```python
from build123d import *

# Parameters (mm, degrees)
SKETCH1_W            = 128
SKETCH1_H            = 85.7
BOSS_EXTRUDE1_DEPTH  = 3
M6_CLEARANCE_HOLE1_D = 6.6
FILLET1_R            = 3


with BuildPart() as part:
    # Sketch1 → Boss-Extrude1 (new body)
    with BuildSketch(Plane(origin=(0, 0, 0), x_dir=(1, 0, 0), z_dir=(0, 1, 0))):
        Rectangle(SKETCH1_W, SKETCH1_H)
    extrude(amount=BOSS_EXTRUDE1_DEPTH)

    # M6 Clearance Hole1 (through all)
    with Locations(Plane(origin=(0, 3, 0), x_dir=(1, 0, 0), z_dir=(0, 1, 0))):
        with Locations((-60.5, 39.35), (0, 39.35), (60.5, 39.35), (60.5, 0), (60.5, -39.35), (0, -39.35), (-60.5, -39.35), (-60.5, 0), (0, -20.01), (0, 20.01)):
            Hole(M6_CLEARANCE_HOLE1_D / 2)

    # Fillet1
    fillet1_edges = [part.edges().sort_by_distance(p)[0] for p in [
        (64, 1.5, 42.85),
        (-64, 1.5, 42.85),
        (-64, 1.5, -42.85),
        (64, 1.5, -42.85),
    ]]
    fillet(fillet1_edges, radius=FILLET1_R)


solid = part.part
```
Read the model definition and answer for the solid it produces. Units are mm, in the model's axes. Give positions to 0.01 mm unless a question says otherwise; leave off trailing zeros. Write each loop counter-clockwise with the first axis right and the second up, starting at its lowest first coordinate (ties: lowest second). Pieces come first, ordered by that corner, then holes. Notation, with made-up numbers: M 78.5,80.25 L 96.5,80.25 A24 ccw 96.5,98.25 Z; hole C 87,50 d8. An arc over 180 degrees is marked long. Put each result on its own line as item: value. Start each with the question number.
1. The part is cut by section A-A, the plane z = 0. Give the vertices of the cut face in (x, y), and give its area (3 significant figures).
2. The part is cut by section C-C, the plane x = 0. Give the vertices of the cut face in (y, z), and give its area (3 significant figures).
3. Consider line 1 along Z through (x, y) = (0, 1.1); line 2 along X through (y, z) = (1.3, -39.35); line 3 along Z through (x, y) = (-60.5, 1.55). Determine where each line is inside the solid, lowest interval first.
4. The part is cut by section B-B, the plane z = 20.01. Give the vertices of the cut face in (x, y).
5. For a pull along X with two mould halves and no side action, classify faces 1 (the cylindrical face through (-63.14, 1.52, -41.95)), 2 (the cylindrical face through (0.72, 1.48, 42.57)), 3 (the cylindrical face through (0.43, 1.48, -42.62)), 4 (the cylindrical face through (63.1, 1.52, 41.99)) as released by +X, released by -X, zero draft, split by the parting line, or undercut.
6. The part is cut by section D-D, the plane y = 1.65. Give the number of separate pieces and of enclosed holes in the cut face, and give its area (3 significant figures).
Final values:
1. outline: M -64,0 L -63.8,0 L -63.8,3 L -64,3 Z; M -57.2,0 L 57.2,0 L 57.2,3 L -57.2,3 Z; M 63.8,0 L 64,0 L 64,3 L 63.8,3 Z
1. area: 344 mm²
2. outline: M 0,-42.85 L 3,-42.85 L 3,-42.65 L 0,-42.65 Z; M 0,-36.05 L 3,-36.05 L 3,-23.31 L 0,-23.31 Z; M 0,-16.71 L 3,-16.71 L 3,16.71 L 0,16.71 Z; M 0,23.31 L 3,23.31 L 3,36.05 L 0,36.05 Z; M 0,42.65 L 3,42.65 L 3,42.85 L 0,42.85 Z
2. area: 178 mm²
3. line 1: z = -42.85 to -42.65, -36.05 to -23.31, -16.71 to 16.71, 23.31 to 36.05, 42.65 to 42.85
3. line 2: x = -64 to -63.8, -57.2 to -3.3, 3.3 to 57.2, 63.8 to 64
3. line 3: z = -42.85 to -42.65, -36.05 to -3.3, 3.3 to 36.05, 42.65 to 42.85
4. outline: M -64,0 L -3.3,0 L -3.3,3 L -64,3 Z; M 3.3,0 L 64,0 L 64,3 L 3.3,3 Z
5. face 1: released by -X
5. face 2: undercut
5. face 3: undercut
5. face 4: released by +X
6. separate pieces: 1
6. enclosed holes: 10
6. area: 10,600 mm²
